```python
from build123d import *

# Parameters (mm, degrees)
SKETCH1_R                            = 6
SKETCH1_R_2                          = 1.35
EIXO_DEPTH                           = 18
SKETCH2_R                            = 1.5
REBAIXO_DE_ENCAIXE_NO_SERVO_DEPTH    = 4
REBAIXO_START                        = -2
SKETCH3_R                            = 3
REBAIXO_DE_ENCAIXE_DO_PARAFUSO_DEPTH = 15.370705544
SKETCH4_R                            = 12
SKETCH4_R_2                          = 3
SKETCH4_R_3                          = 1
CORPO_DE_FIXA_O_NO_ANTEBRA_O_DEPTH   = 3
RAIO_DE_AL_VIO_0_5MM_R               = 0.5
CHANFROS_0_5MM_SIZE                  = 0.5
ENCAIXE_DA_ENGRENAGEM_DO_SERVO_DEPTH = 4


with BuildPart() as part:
    # Sketch1 → Eixo (new body)
    with BuildSketch(Plane(origin=(0, 0, 0), x_dir=(1, 0, 0), z_dir=(0, 1, 0))):
        with Locations(Location((0, 0, 0), (0, 0, 270))):
            Circle(SKETCH1_R)
        with Locations(Location((0, 0, 0), (0, 0, 270))):
            Circle(SKETCH1_R_2, mode=Mode.SUBTRACT)
    extrude(amount=EIXO_DEPTH)

    # Sketch2 → Rebaixo de Encaixe no Servo (cut)
    with BuildSketch(Plane.XZ):
        with Locations(Location((0, 0, 0), (0, 0, 270))):
            Circle(SKETCH2_R)
    extrude(amount=-REBAIXO_DE_ENCAIXE_NO_SERVO_DEPTH, mode=Mode.SUBTRACT)

    # Sketch3 → Rebaixo de Encaixe do Parafuso (cut, through all)
    with BuildSketch(Plane.XZ.offset(-4).offset(REBAIXO_START)):
        with Locations(Location((0, 0, 0), (0, 0, 270))):
            Circle(SKETCH3_R)
    extrude(amount=-REBAIXO_DE_ENCAIXE_DO_PARAFUSO_DEPTH, mode=Mode.SUBTRACT)

    # Sketch4 → Corpo de Fixação no Antebraço (add)
    with BuildSketch(Plane(origin=(0, 18, 0), x_dir=(1, 0, 0), z_dir=(0, 1, 0))):
        with Locations(Location((0, 0, 0), (0, 0, 270))):
            Circle(SKETCH4_R)
        with Locations(Location((0, 0, 0), (0, 0, 90))):
            Circle(SKETCH4_R_2, mode=Mode.SUBTRACT)
        with Locations(Location((0, 9.375, 0), (0, 0, 270))):
            Circle(SKETCH4_R_3, mode=Mode.SUBTRACT)
        with Locations(Location((9.375, 0, 0), (0, 0, 270))):
            Circle(SKETCH4_R_3, mode=Mode.SUBTRACT)
        with Locations(Location((0, -9.375, 0), (0, 0, 270))):
            Circle(SKETCH4_R_3, mode=Mode.SUBTRACT)
        with Locations(Location((-9.375, 0, 0), (0, 0, 270))):
            Circle(SKETCH4_R_3, mode=Mode.SUBTRACT)
    extrude(amount=CORPO_DE_FIXA_O_NO_ANTEBRA_O_DEPTH)

    # Raio de Alívio - 0.5mm
    raio_de_al_vio_0_5mm_edges = [part.edges().sort_by_distance(p)[0] for p in [
        (0, 18, -6),
    ]]
    fillet(raio_de_al_vio_0_5mm_edges, radius=RAIO_DE_AL_VIO_0_5MM_R)

    # Chanfros 0.5mm
    chanfros_0_5mm_edges = [part.edges().sort_by_distance(p)[0] for p in [
        (0, 0, -6),
        (0, 21, -12),
        (0, 18, -12),
    ]]
    chamfer(chanfros_0_5mm_edges, length=CHANFROS_0_5MM_SIZE)

    # Sketch6 → Encaixe da Engrenagem do Servo (cut)
    with BuildSketch(Plane.XZ):
        with BuildLine():
            Line((-1.674039734, -1.856768959), (-1.692843967, -2.385352029))
            ThreePointArc((-1.692843967, -2.385352029), (-1.670905751, -2.400770495), (-1.648827112, -2.415987201))
            Line((-1.648827112, -2.415987201), (-1.159687035, -2.214751901))
            Line((-1.159687035, -2.214751901), (-1.046447234, -2.731404984))
            ThreePointArc((-1.046447234, -2.731404984), (-1.02136383, -2.740883238), (-0.996194592, -2.750131149))
            Line((-0.996194592, -2.750131149), (-0.572466934, -2.433573835))
            Line((-0.572466934, -2.433573835), (-0.334298372, -2.905833718))
            ThreePointArc((-0.334298372, -2.905833718), (-0.307645864, -2.908776207), (-0.280967502, -2.911474242))
            Line((-0.280967502, -2.911474242), (0.05072337, -2.499485375))
            Line((0.05072337, -2.499485375), (0.398855685, -2.897678233))
            ThreePointArc((0.398855685, -2.897678233), (0.425402623, -2.893900069), (0.45191381, -2.889878701))
            Line((0.45191381, -2.889878701), (0.670726538, -2.408345057))
            Line((0.670726538, -2.408345057), (1.106948173, -2.707450968))
            ThreePointArc((1.106948173, -2.707450968), (1.131721499, -2.697189546), (1.156399715, -2.686701453))
            Line((1.156399715, -2.686701453), (1.248585491, -2.165879561))
            Line((1.248585491, -2.165879561), (1.745487037, -2.3471046))
            ThreePointArc((1.745487037, -2.3471046), (1.766930151, -2.331004685), (1.788224772, -2.314708872))
            Line((1.788224772, -2.314708872), (1.747991225, -1.787323887))
            Line((1.747991225, -1.787323887), (2.27435053, -1.839281019))
            ThreePointArc((2.27435053, -1.839281019), (2.291116083, -1.818354227), (2.307689091, -1.79727462))
            Line((2.307689091, -1.79727462), (2.137564242, -1.29646408))
            Line((2.137564242, -1.29646408), (2.660308215, -1.215888647))
            ThreePointArc((2.660308215, -1.215888647), (2.671342766, -1.191449885), (2.682152817, -1.166910993))
            Line((2.682152817, -1.166910993), (2.392826237, -0.724142666))
            Line((2.392826237, -0.724142666), (2.879108951, -0.51609752))
            ThreePointArc((2.879108951, -0.51609752), (2.883719158, -0.489682365), (2.888087017, -0.463226057))
            Line((2.888087017, -0.463226057), (2.497738158, -0.106320706))
            Line((2.497738158, -0.106320706), (2.917004683, 0.216121913))
            ThreePointArc((2.917004683, 0.216121913), (2.91490087, 0.242853699), (2.912552089, 0.269565076))
            Line((2.912552089, 0.269565076), (2.445708005, 0.518181775))
            Line((2.445708005, 0.518181775), (2.771614282, 0.934761611))
            ThreePointArc((2.771614282, 0.934761611), (2.76292864, 0.960130372), (2.754010801, 0.985418444))
            Line((2.754010801, 0.985418444), (2.240005024, 1.11012499))
            Line((2.240005024, 1.11012499), (2.452073163, 1.594666799))
            ThreePointArc((2.452073163, 1.594666799), (2.437351442, 1.617078523), (2.422424885, 1.639354347))
            Line((2.422424885, 1.639354347), (1.893554289, 1.632314968))
            Line((1.893554289, 1.632314968), (1.97845927, 2.154373208))
            ThreePointArc((1.97845927, 2.154373208), (1.958626489, 2.172419682), (1.938629106, 2.190283587))
            Line((1.938629106, 2.190283587), (1.428124573, 2.051940594))
            Line((1.428124573, 2.051940594), (1.380531504, 2.578712424))
            ThreePointArc((1.380531504, 2.578712424), (1.356833831, 2.591259724), (1.333022129, 2.603589254))
            Line((1.333022129, 2.603589254), (0.872960539, 2.342635246))
            Line((0.872960539, 2.342635246), (0.695859866, 2.841021655))
            ThreePointArc((0.695859866, 2.841021655), (0.669786312, 2.847281387), (0.64365647, 2.853301833))
            Line((0.64365647, 2.853301833), (0.262945183, 2.48613351))
            Line((0.262945183, 2.48613351), (-0.032535206, 2.924819047))
            ThreePointArc((-0.032535206, 2.924819047), (-0.059346343, 2.924397889), (-0.086152492, 2.923730964))
            Line((-0.086152492, 2.923730964), (-0.363591985, 2.473418862))
            Line((-0.363591985, 2.473418862), (-0.758885972, 2.824839302))
            ThreePointArc((-0.758885972, 2.824839302), (-0.784750049, 2.817763716), (-0.810548177, 2.810451326))
            Line((-0.810548177, 2.810451326), (-0.967283332, 2.305290211))
            Line((-0.967283332, 2.305290211), (-1.437553141, 2.547364514))
            ThreePointArc((-1.437553141, 2.547364514), (-1.460845024, 2.534079086), (-1.484014138, 2.520580694))
            Line((-1.484014138, 2.520580694), (-1.51019671, 1.992311697))
            Line((-1.51019671, 1.992311697), (-2.025893559, 2.109829445))
            ThreePointArc((-2.025893559, 2.109829445), (-2.045149734, 2.091168948), (-2.064234034, 2.072332708))
            Line((-2.064234034, 2.072332708), (-1.958218874, 1.554148912))
            Line((-1.958218874, 1.554148912), (-2.486939634, 1.539726033))
            ThreePointArc((-2.486939634, 1.539726033), (-2.500950163, 1.516862973), (-2.514750513, 1.493872437))
            Line((-2.514750513, 1.493872437), (-2.283198945, 1.018333235))
            Line((-2.283198945, 1.018333235), (-2.791722146, 0.872875971))
            ThreePointArc((-2.791722146, 0.872875971), (-2.799606697, 0.84724692), (-2.807255969, 0.821546666))
            Line((-2.807255969, 0.821546666), (-2.464717229, 0.418531936))
            Line((-2.464717229, 0.418531936), (-2.921090488, 0.151179902))
            ThreePointArc((-2.921090488, 0.151179902), (-2.922353645, 0.124395226), (-2.923371208, 0.097600096))
            Line((-2.923371208, 0.097600096), (-2.491368265, -0.207567264))
            Line((-2.491368265, -0.207567264), (-2.866915971, -0.580015356))
            ThreePointArc((-2.866915971, -0.580015356), (-2.861478366, -0.606272677), (-2.855800283, -0.632479046))
            Line((-2.855800283, -0.632479046), (-2.36147747, -0.82062425))
            Line((-2.36147747, -0.82062425), (-2.632602581, -1.274766117))
            ThreePointArc((-2.632602581, -1.274766117), (-2.620805878, -1.298846238), (-2.608788923, -1.322817204))
            Line((-2.608788923, -1.322817204), (-2.083206361, -1.382118395))
            Line((-2.083206361, -1.382118395), (-2.232873088, -1.889418634))
            ThreePointArc((-2.232873088, -1.889418634), (-2.215458518, -1.909808513), (-2.19785776, -1.930037892))
            Line((-2.19785776, -1.930037892), (-1.674039734, -1.856768959))
        make_face()
    extrude(amount=-ENCAIXE_DA_ENGRENAGEM_DO_SERVO_DEPTH, mode=Mode.SUBTRACT)


solid = part.part
```
For this review, take the finished solid that the model builds, in its own axes (mm). A direction names the side the tool comes from. Give positions to 0.01 mm unless a question says otherwise; leave off trailing zeros. Loops run counter-clockwise (first coordinate to the right, second up) from the corner with the lowest first, then second, coordinate; pieces in that order, holes last. Notation, with made-up numbers: M 70.5,73 L 108.5,73 A21 ccw 108.5,108 Z; hole C 13.25,62.25 d3. An arc over 180 degrees is marked long. One line per item, written item: value. Start each with the question number.
Q1. Add section A-A (y = 16.25). Give the boundary of the cut face in (x, z), and give its area (3 significant figures).
Q2. Draft analysis for pull direction Z (two halves, no side actions). For faces 4 (the face through (-1, 0, -3)), 5 (the face through (3.604, 19.486, 11.446)), 6 (the face through (-0.608, 19.479, 8.581)), 7 (the face through (-0.887, 19.479, -8.914)), state which applies: released by +Z, released by -Z, zero draft, split by the parting line, or undercut.
Q3. Clearance check with flat-ended pins moving along their axes: pin 1 Ø1.8 at (x, z) = (0, 9.375) entering from -Y; pin 2 Ø8 at (y, z) = (9, -8) entering from -X; pin 3 Ø12 at (x, y) = (0.5, 3.5) entering from -Z; pin 4 Ø3 at (x, z) = (0, -9.375) entering from +Y. State where each tip first meets the part, or that it passes through.
Q4. For L1, parallel to X at y = 19.65, z = 0 (3 decimals); L2, parallel to Y at x = 1.25, z = -1; L3, parallel to Y at x = -7, z = 2.5, list the stretches that pass through material, from the lowest coordinate up.
Q5. Machinability: for faces 1 (the face through (0.406, 4.986, 1.288)), 2 (the face through (-5, 18, 5)), 3 (the face through (-0.9, 13.4, -2.86)), which of the approach directions +Z, -Z, +X, -X, +Y, -Y give a long, thin tool a straight path to every point of the face, cutting with its end or side? Answer none if there is none.
Reply:
1. outline: C 0,0 d12; hole C 0,0 d6
1. area: 84.8 mm²
2. face 4: zero draft
2. face 5: split by the parting line
2. face 6: undercut
2. face 7: undercut
3. pin 1: through
3. pin 2: x = -4.47
3. pin 3: z = -6
3. pin 4: y = 21
4. L1: -12 to -10.375, -8.375 to -3, 3 to 8.375, 10.375 to 12
4. L2: 4 to 6
4. L3: 18 to 21
5. face 1: +Y, -Y
5. face 2: -Y
5. face 3: +Y
